Geometry: final body of the model. Coordinates: model frame, mm. A direction names the side the tool comes from. Round coordinates to 2 decimals unless told otherwise and drop trailing zeros. Loops run counter-clockwise (first coordinate to the right, second up) from the corner with the lowest first, then second, coordinate; pieces in that order, holes last. Notation, with made-up numbers: (17.5, 89.25) - (36.5, 89.25) arc R27 ccw to (36.5, 107.25) - close; hole circle Ø5 at (28.25, 46.25). An arc over 180 degrees is marked (long way). Answer as a JSON object with one key per item and string values. Group by question number.
Item 1: Section C-C (z = -14.5). Return the cut outline in (x, y).
Item 2: Section B-B (x = 5.5). Return the cut outline in (y, z), plus the area to 3 significant figures.
Item 3: Section A-A (y = 32.25). Return the cut outline in (x, z).
Item 4: First-contact query: pin 1 (7.5 mm diameter, centred on x = -6, y = 31, fed in from -Z); pin 2 (0.9 mm diameter, centred on x = -5, y = 30.5, fed in from -Z); pin 3 (1.4 mm diameter, centred on x = 5.5, y = 30, fed in from -Z). Flat tips, straight axial feed; report the tip coordinate or a pass-through.
Item 5: Line query: line 1 (Y direction, x = 5.5, z = -10.65); line 2 (Y direction, x = 5, z = -11.25); line 3 (Z direction, x = 7.5, y = 32.5). Output: solid intervals per line, ascending.
Item 6: Section D-D (x = -1.25). Return the cut outline in (y, z), plus the area to 3 significant figures.
Item 7: Reachability of faces 4 (the face through (-6.4, 30, -10.2)), 5 (the face through (5.45, 30.21, -7.06)), 6 (the face through (7, 30, -11.456)), 7 (the face through (-7, 30, -11.456)) from +Z, -Z, +X, -X, +Y, -Y: full face, straight path, thin tool, end or side. Return the list, or none.
Item 8: Draft query along Y for faces 1 (the face through (0, 15, -9)), 2 (the face through (-6, 30, -9)), 3 (the face through (-2, 30.2, -13.4)). Return one class per face: released by +Y, released by -Y, zero draft, split by the parting line, or undercut.
```python
from build123d import *

# Parameters (mm, degrees)
PAD005_DEPTH    = 30
PAD006_DEPTH    = 30
SKETCH043_R     = 0.9
POCKET016_DEPTH = 5


with BuildPart() as part:
    # Sketch037 → Pad005 (new body)
    with BuildSketch(Plane.XZ.offset(-45)):
        with BuildLine():
            ThreePointArc((-10.178404, -6.708561), (-5.503497, -7.075491), (-1.569892, -4.522816))
            ThreePointArc((1.569892, -4.522816), (0, -3.761944), (-1.569892, -4.522816))
            ThreePointArc((1.569892, -4.522816), (5.517054, -7.07892), (10.204085, -6.697484))
            ThreePointArc((10.902995, -7.156215), (10.677354, -6.738211), (10.204085, -6.697484))
            Line((10.902995, -11.456215), (10.902995, -7.156215))
            Line((10.902995, -11.456215), (-10.875555, -11.456215))
            Line((-10.875555, -11.456215), (-10.875555, -7.168051))
            ThreePointArc((-10.178404, -6.708561), (-10.650714, -6.750574), (-10.875555, -7.168051))
        make_face()
    extrude(amount=PAD005_DEPTH)

    # Sketch042 → Pad006 (join)
    with BuildSketch(Plane.XZ.offset(-45)):
        Polygon((-4, -11.4), (0, -15.4), (4, -11.4), align=None)
    extrude(amount=PAD006_DEPTH)

    # Sketch043 → Pocket016 (cut)
    with BuildSketch(Plane.XY.offset(-9)):
        with Locations((-5.5, 30)):
            Circle(SKETCH043_R)
        with Locations((-5.5, -30)):
            Circle(SKETCH043_R)
        with Locations((5.5, 30)):
            Circle(SKETCH043_R)
        with Locations((5.5, -30)):
            Circle(SKETCH043_R)
    extrude(amount=-POCKET016_DEPTH, mode=Mode.SUBTRACT)


solid = part.part
```
Values:
{
 "1": {"outline": "(-0.9, 15) - (0.9, 15) - (0.9, 45) - (-0.9, 45) - close"},
 "2": {"outline": "(15, -11.46) - (29.1, -11.46) - (29.1, -9) - (30.9, -9) - (30.9, -11.46) - (45, -11.46) - (45, -7.07) - (15, -7.07) - close", "area": "127 mm^2"},
 "3": {"outline": "(-10.88, -11.46) - (-3.94, -11.46) - (0, -15.4) - (3.94, -11.46) - (10.9, -11.46) - (10.9, -7.16) arc R0.5 ccw to (10.2, -6.7) arc R7.3 cw to (1.57, -4.52) arc R2 ccw to (-1.57, -4.52) arc R7.3 cw to (-10.18, -6.71) arc R0.5 ccw to (-10.88, -7.17) - close"},
 "4": {"pin 1": "stops at z = -13.15", "pin 2": "stops at z = -11.46", "pin 3": "stops at z = -9"},
 "5": {"line 1": "y = 15 to 29.1, 30.9 to 45", "line 2": "y = 15 to 29.25, 30.75 to 45", "line 3": "z = -11.46 to -7.3"},
 "6": {"outline": "(15, -14.15) - (45, -14.15) - (45, -4.2) - (15, -4.2) - close", "area": "298 mm^2"},
 "7": {"face 4": "-Z", "face 5": "+Z, +Y, -Y", "face 6": "-Z, +X, +Y, -Y", "face 7": "-Z, -X, +Y, -Y"},
 "8": {"face 1": "released by -Y", "face 2": "undercut", "face 3": "zero draft"}
}
